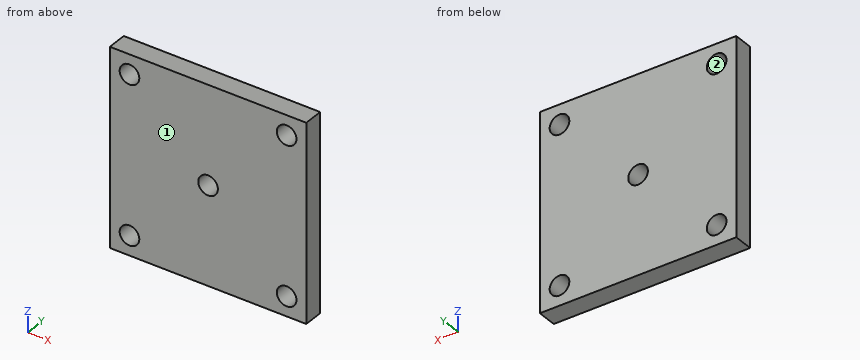
from build123d import *

# Parameters (mm, degrees)
F0_W     = 60
F0_H     = 60
F0_R     = 3
F1_DEPTH = 6


with BuildPart() as f1:
    # F0 (on Front) → F1 (new body)
    with BuildSketch(Plane.XZ):
        Rectangle(F0_W, F0_H)
        with Locations((-24, -24)):
            Circle(F0_R, mode=Mode.SUBTRACT)
        with Locations((24, -24)):
            Circle(F0_R, mode=Mode.SUBTRACT)
        with Locations((-24, 24)):
            Circle(F0_R, mode=Mode.SUBTRACT)
        Circle(F0_R, mode=Mode.SUBTRACT)
        with Locations((24, 24)):
            Circle(F0_R, mode=Mode.SUBTRACT)
    extrude(amount=F1_DEPTH)


solid = f1.part
Geometry check sheet. Reference: the model listing, model coordinates, mm. Face numbers are marked on the shaded views. Give positions to 0.01 mm unless a question says otherwise; leave off trailing zeros. Loops run counter-clockwise (first coordinate to the right, second up) from the corner with the lowest first, then second, coordinate; pieces in that order, holes last. Notation, with made-up numbers: M 24.5,86 L 42.5,86 A27 ccw 42.5,120 Z; hole C 36.25,44.25 d1. An arc over 180 degrees is marked long. Answer as a JSON object with one key per item and string values. Group by question number.
Item 1: Sectioned sample at D-D on x = 2. Record the boundary of the cut face in (y, z), plus the area to 3 significant figures.
Item 2: Sectioned sample at B-B on z = 24. Record the boundary of the cut face in (x, y).
Item 3: Sectioned sample at C-C on y = -0.9. Record the boundary of the cut face in (x, z), plus the area to 3 significant figures.
Item 4: Material ranges on L1, parallel to Z at x = -24, y = -3.4; L2, parallel to X at y = -3.9, z = 23.5; L3, parallel to X at y = -4.85, z = -0.5, recorded low to high.
Item 5: Sectioned sample at A-A on x = -24. Record the boundary of the cut face in (y, z), plus the area to 3 significant figures.
Item 6: Mould release check, pull along Z, two halves, no side actions. Record for the marked faces 1 and 2: pulls with the +Z half, pulls with the -Z half, needs draft (parallel to the pull), parting line crosses it, or undercut.
Findings below:
{
 "1": {"outline": "M -6,-30 L 0,-30 L 0,-2.24 L -6,-2.24 Z; M -6,2.24 L 0,2.24 L 0,30 L -6,30 Z", "area": "333 mm2"},
 "2": {"outline": "M -30,-6 L -27,-6 L -27,0 L -30,0 Z; M -21,-6 L 21,-6 L 21,0 L -21,0 Z; M 27,-6 L 30,-6 L 30,0 L 27,0 Z"},
 "3": {"outline": "M -30,-30 L 30,-30 L 30,30 L -30,30 Z; hole C -24,-24 d6; hole C -24,24 d6; hole C 0,0 d6; hole C 24,-24 d6; hole C 24,24 d6", "area": "3,460 mm2"},
 "4": {"L1": "-30 to -27, -21 to 21, 27 to 30", "L2": "-30 to -26.96, -21.04 to 21.04, 26.96 to 30", "L3": "-30 to -2.96, 2.96 to 30"},
 "5": {"outline": "M -6,-30 L 0,-30 L 0,-27 L -6,-27 Z; M -6,-21 L 0,-21 L 0,21 L -6,21 Z; M -6,27 L 0,27 L 0,30 L -6,30 Z", "area": "288 mm2"},
 "6": {"face 1": "needs draft", "face 2": "undercut"}
}
